```python
from build123d import *

# Parameters (mm, degrees)
CUT_EXTRUDE1_REACH = 71.527
SKETCH2_R          = 4.5


with BuildPart() as part:
    # Sketch1 → Revolve1 (revolve)
    with BuildSketch(Plane.XY, mode=Mode.PRIVATE) as revolve1_sk:
        Polygon((-45, 28), (-45, 22), (-29.5, 22), (-29.5, 20.5), (-31, 20.5), (-31, 0), (-26, 0), (-22.649787367, 19), (-15, 19), (-15, 21), (-20, 21), (-20, 26), (-15, 26), (-15, 28), (-29, 28), align=None)
    revolve(revolve1_sk.sketch.rotate(Axis((0, 30.618797564, 0), (0, -1, 0)), 270), axis=Axis((0, 30.618797564, 0), (0, -1, 0)))

    # Sketch2 → Cut-Extrude1 (cut, up to next)
    with BuildSketch(Plane(origin=(0, 28, 0), x_dir=(1, 0, 0), z_dir=(0, 1, 0)), mode=Mode.PRIVATE) as cut_extrude1_sk1:
        with Locations(Location((0, 37, 0), (0, 0, 270))):
            Circle(SKETCH2_R)
    cut_extrude1_tool1 = extrude(cut_extrude1_sk1.sketch, amount=-CUT_EXTRUDE1_REACH, mode=Mode.PRIVATE) & part.part
    # Sketch2 → Cut-Extrude1 (cut, up to next)
    with BuildSketch(Plane(origin=(0, 28, 0), x_dir=(1, 0, 0), z_dir=(0, 1, 0)), mode=Mode.PRIVATE) as cut_extrude1_sk2:
        with Locations(Location((32.04293994, 18.5, 0), (0, 0, 270))):
            Circle(SKETCH2_R)
    cut_extrude1_tool2 = extrude(cut_extrude1_sk2.sketch, amount=-CUT_EXTRUDE1_REACH, mode=Mode.PRIVATE) & part.part
    # Sketch2 → Cut-Extrude1 (cut, up to next)
    with BuildSketch(Plane(origin=(0, 28, 0), x_dir=(1, 0, 0), z_dir=(0, 1, 0)), mode=Mode.PRIVATE) as cut_extrude1_sk3:
        with Locations(Location((32.04293994, -18.5, 0), (0, 0, 270))):
            Circle(SKETCH2_R)
    cut_extrude1_tool3 = extrude(cut_extrude1_sk3.sketch, amount=-CUT_EXTRUDE1_REACH, mode=Mode.PRIVATE) & part.part
    # Sketch2 → Cut-Extrude1 (cut, up to next)
    with BuildSketch(Plane(origin=(0, 28, 0), x_dir=(1, 0, 0), z_dir=(0, 1, 0)), mode=Mode.PRIVATE) as cut_extrude1_sk4:
        with Locations(Location((0, -37, 0), (0, 0, 270))):
            Circle(SKETCH2_R)
    cut_extrude1_tool4 = extrude(cut_extrude1_sk4.sketch, amount=-CUT_EXTRUDE1_REACH, mode=Mode.PRIVATE) & part.part
    # Sketch2 → Cut-Extrude1 (cut, up to next)
    with BuildSketch(Plane(origin=(0, 28, 0), x_dir=(1, 0, 0), z_dir=(0, 1, 0)), mode=Mode.PRIVATE) as cut_extrude1_sk5:
        with Locations(Location((-32.04293994, -18.5, 0), (0, 0, 270))):
            Circle(SKETCH2_R)
    cut_extrude1_tool5 = extrude(cut_extrude1_sk5.sketch, amount=-CUT_EXTRUDE1_REACH, mode=Mode.PRIVATE) & part.part
    # Sketch2 → Cut-Extrude1 (cut, up to next)
    with BuildSketch(Plane(origin=(0, 28, 0), x_dir=(1, 0, 0), z_dir=(0, 1, 0)), mode=Mode.PRIVATE) as cut_extrude1_sk6:
        with Locations(Location((-32.04293994, 18.5, 0), (0, 0, 270))):
            Circle(SKETCH2_R)
    cut_extrude1_tool6 = extrude(cut_extrude1_sk6.sketch, amount=-CUT_EXTRUDE1_REACH, mode=Mode.PRIVATE) & part.part
    add(cut_extrude1_tool1.solids().sort_by_distance((0, 28, -37))[0], mode=Mode.SUBTRACT)
    add(cut_extrude1_tool2.solids().sort_by_distance((32.04294, 28, -18.5))[0], mode=Mode.SUBTRACT)
    add(cut_extrude1_tool3.solids().sort_by_distance((32.04294, 28, 18.5))[0], mode=Mode.SUBTRACT)
    add(cut_extrude1_tool4.solids().sort_by_distance((0, 28, 37))[0], mode=Mode.SUBTRACT)
    add(cut_extrude1_tool5.solids().sort_by_distance((-32.04294, 28, 18.5))[0], mode=Mode.SUBTRACT)
    add(cut_extrude1_tool6.solids().sort_by_distance((-32.04294, 28, -18.5))[0], mode=Mode.SUBTRACT)


solid = part.part
```
Geometry: final body of the model. Coordinates: model frame, mm. A direction names the side the tool comes from. Give positions to 0.01 mm unless a question says otherwise; leave off trailing zeros. Order: outer loops, then holes, each group sorted by start corner. A loop starts at its lowest first (then second) coordinate and runs counter-clockwise, first axis right, second up. Notation, with made-up numbers: (33, 20) -> (61, 20) arc R10 ccw to (61, 36) -> close; hole circle Ø1 at (30.5, 64.25). An arc over 180 degrees is marked (long way). Write each question's results on one line, items separated by ' | '. Start each with the question number.
1) First-contact query: pin 1 (3 mm diameter, centred on x = 14.5, y = 5.5, fed in from -Z); pin 2 (3 mm diameter, centred on y = 15, z = 3.5, fed in from -X); pin 3 (6 mm diameter, centred on x = 26.5, y = 14.5, fed in from -Z). Flat tips, straight axial feed; report the tip coordinate or a pass-through.
2) Section D-D (y = 15.5). Return loops of the section in (x, z), then the cut area to 3 significant figures.
3) Line query: line 1 (X direction, y = 24.95, z = 0); line 2 (Y direction, x = -16, z = -3.5); line 3 (Z direction, x = 35.5, y = 22.5). Output: solid intervals per line, ascending. Write a range as from..to.
4) Set-up query: faces 4 (the cylindrical face through (-0.66, 20.014, -14.985)), 5 (the flat face through (5, 19, 15)), 6 (the cylindrical face through (19.524, 23.535, -4.336)). Return all of +Z, -Z, +X, -X, +Y, -Y with unobstructed straight access to the full face (end or side cutting, diameter ignored); none if empty.
5) Section C-C (z = 18.5). Count the separate pieces of the cut face and the enclosed holes in it, then the cut area to 3 significant figures.
6) Draft query along X for faces 1 (the flat face through (11.34, 20.5, -27.41)), 2 (the cylindrical face through (-8.86, 21.24, 28.14)), 3 (the flat face through (-15, 26, 3)). Return one class per face: pulls with the +X half, pulls with the -X half, needs draft (parallel to the pull), parting line crosses it, or undercut.
7) Section A-A (z = 0). Return loops of the section in (x, y), then the cut area to 3 significant figures.
8) Section B-B (x = 34). Return loops of the section in (y, z).
Calculated:
1) pin 1: z = -28.14 | pin 2: x = -30.94 | pin 3: z = -20.22
2) outline: circle Ø62 at (0, 0); hole circle Ø46.53 at (0, 0) | area: 1,320 mm2
3) line 1: -45..-20, 20..45 | line 2: 19..21, 26..28 | line 3: -27.65..-21.38, -15.62..15.62, 21.38..27.65
4) face 4: +Y, -Y | face 5: -Y | face 6: none
5) separate pieces: 3 | enclosed holes: 1 | area: 798 mm2
6) face 1: needs draft | face 2: parting line crosses it | face 3: undercut
7) outline: (-45, 22) -> (-29.5, 22) -> (-29.5, 20.5) -> (-31, 20.5) -> (-31, 0) -> (-26, 0) -> (-22.65, 19) -> (-15, 19) -> (-15, 21) -> (-20, 21) -> (-20, 26) -> (-15, 26) -> (-15, 28) -> (-45, 28) -> close; (15, 19) -> (22.65, 19) -> (26, 0) -> (31, 0) -> (31, 20.5) -> (29.5, 20.5) -> (29.5, 22) -> (45, 22) -> (45, 28) -> (15, 28) -> (15, 26) -> (20, 26) -> (20, 21) -> (15, 21) -> close | area: 655 mm2
8) outline: (22, -29.48) -> (28, -29.48) -> (28, -22.55) -> (22, -22.55) -> close; (22, -14.45) -> (28, -14.45) -> (28, 14.45) -> (22, 14.45) -> close; (22, 22.55) -> (28, 22.55) -> (28, 29.48) -> (22, 29.48) -> close
